from build123d import *

# Parameters (mm, degrees)
SKETCH_2_R      = 2.65
SKETCH_2_R_2    = 1.65
SKETCH_2_R_3    = 10
EXTRUDE_1_DEPTH = 4


with BuildPart() as part:
    # 草图2 → 凸台-拉伸1 (new body)
    with BuildSketch(Plane.XY):
        Polygon((80, 100), (-26.410161514, 100), (-80, -100), (80, -100), align=None)
        with Locations((-65, -87)):
            Circle(SKETCH_2_R, mode=Mode.SUBTRACT)
        with Locations((-15, -87)):
            Circle(SKETCH_2_R, mode=Mode.SUBTRACT)
        with Locations((-9, -30)):
            Circle(SKETCH_2_R_2, mode=Mode.SUBTRACT)
        with Locations((35, -87)):
            Circle(SKETCH_2_R, mode=Mode.SUBTRACT)
        with Locations((-9, 10)):
            Circle(SKETCH_2_R_2, mode=Mode.SUBTRACT)
        with Locations((-9, 50)):
            Circle(SKETCH_2_R_2, mode=Mode.SUBTRACT)
        with Locations((20.5, 75)):
            Circle(SKETCH_2_R_2, mode=Mode.SUBTRACT)
        with Locations((35.5, 75)):
            Circle(SKETCH_2_R_2, mode=Mode.SUBTRACT)
        with Locations((64, 80)):
            Circle(SKETCH_2_R_3, mode=Mode.SUBTRACT)
    extrude(amount=EXTRUDE_1_DEPTH)


solid = part.part
Can you work these out from the model? Positions are in its coordinate system, mm. Coordinates: 2 decimals unless noted, no trailing zeros. Loops run counter-clockwise (first coordinate to the right, second up) from the corner with the lowest first, then second, coordinate; pieces in that order, holes last. Notation, with made-up numbers: M 28,12 L 32,12 A27 ccw 32,31 Z; hole C 16.25,61 d1. An arc over 180 degrees is marked long. Return JSON: item names as keys, results as strings. Group by question number.
Item 1: Imagine slicing it at C-C (y = 80). Please give me the cut outline in (x, z).
Item 2: Thinking about a two-plate mould opening in Y: for faces 1 (the cylindrical face through (-63.777, -89.351, 1.972)), 2 (the flat face through (-1, -100, 2)), 3 (the flat face through (17, 1, 0)), which applies, released by +Y, released by -Y, zero draft, split by the parting line, or undercut?
Item 3: I'm going to push flat-ended pins straight in: pin 1 Ø2 at (x, y) = (-9, -30) entering from -Z; pin 2 Ø5.5 at (x, y) = (35.5, 75) entering from -Z; pin 3 Ø2 at (y, z) = (7, 1) entering from -X. Where does each tip first touch, or does it pass through?
Item 4: Imagine slicing it at A-A (x = 64). Please give me the cut outline in (y, z).
Item 5: Imagine slicing it at B-B (z = 1). Give the number of separate pieces and of enclosed holes in the cut face, and give its area (3 significant figures).
Item 6: If I drill on L1, parallel to Y at x = -9, z = 2.1; L2, parallel to Y at x = 64, z = 2.35; L3, parallel to X at y = 75, z = 1.7, over which ranges is the centre line in solid material (lowest first)? Write a range as from..to.
Item 7: Imagine slicing it at D-D (y = 30). Please give me the cut outline in (x, z), and give its area (3 significant figures).
Verdict:
{
 "1": {"outline": "M -31.77,0 L 54,0 L 54,4 L -31.77,4 Z; M 74,0 L 80,0 L 80,4 L 74,4 Z"},
 "2": {"face 1": "undercut", "face 2": "released by -Y", "face 3": "zero draft"},
 "3": {"pin 1": "passes through", "pin 2": "stops at z = 0", "pin 3": "stops at x = -51.6"},
 "4": {"outline": "M -100,0 L 70,0 L 70,4 L -100,4 Z; M 90,0 L 100,0 L 100,4 L 90,4 Z"},
 "5": {"separate pieces": "1", "enclosed holes": "9", "area": "26,200 mm^2"},
 "6": {"L1": "y = -100..-31.65, -28.35..8.35, 11.65..48.35, 51.65..100", "L2": "y = -100..70, 90..100", "L3": "x = -33.11..18.85, 22.15..33.85, 37.15..55.34, 72.66..80"},
 "7": {"outline": "M -45.17,0 L 80,0 L 80,4 L -45.17,4 Z", "area": "501 mm^2"}
}
